Source: CAD feature listing. Evaluate the final solid. Frame: model axes, mm. Give positions to 0.01 mm unless a question says otherwise; leave off trailing zeros. Order: outer loops, then holes, each group sorted by start corner. A loop starts at its lowest first (then second) coordinate and runs counter-clockwise, first axis right, second up. Notation, with made-up numbers: (0, 71.5) -> (26, 71.5) arc R14 cw to (26, 79.5) -> close; hole circle Ø4 at (-36, 69.25). An arc over 180 degrees is marked (long way). Answer in a Markdown table with one row per item.
Autodesk Inventor part; units mm, degrees
ref_plane "YZ Plane" through (0, 0, 0) normal (1, 0, 0) x (0, 1, 0)
ref_plane "XZ Plane" through (0, 0, 0) normal (0, 1, 0) x (-1, 0, 0)
ref_plane "XY Plane" through (0, 0, 0) normal (0, 0, 1) x (1, 0, 0)
sketch "Skizze1" plane through (0, 0, 0) normal (0, 0, 1) x (1, 0, 0)
  line L0 (0, 78) -> (0, -13)
  line L1 (-15, 0) -> (90, 0)
  line L2 (0, 0) -> (75, 0)
  line L3 (75, 0) -> (75, 35)
  line L4 (75, 35) -> (0, 35)
  line L5 (0, 35) -> (0, 0)
  arc A0 (24, 35) -> (56, 35) centre (40, 65) ccw
  dimension "d0" = 75
  dimension "d1" = 35
  dimension "d3" = 35
  dimension "d4" = 30
  dimension "d6" = 34
extrude "Extrusion1" add sketch "Skizze1" along normal blind 2 contours L4 A0 L3 L1 L0
sketch "Skizze2" plane through (0, 0, 2) normal (0, 0, 1) x (1, 0, 0)
  line L0 (36, 6) -> (57, 6)
  line L1 (57, 6) -> (57, 27)
  line L2 (57, 27) -> (36, 27)
  line L3 (36, 27) -> (36, 6)
  line L4 (36, 6) -> (57, 27) construction
  line L5 (57, 6) -> (36, 27) construction
  line L6 (57, 27) -> (15, 27)
  line L7 (15, 27) -> (15, 6)
  line L8 (15, 6) -> (57, 6)
  line L9 (57, 6) -> (57, 27)
  line L10 (75, 0) -> (75, 35)
  line L11 (24, 35) -> (0, 35)
  circle A0 centre (61.35, 21.5) radius 2.25
  circle A1 centre (61.35, 11.5) radius 2.25
  circle A2 centre (11.85, 11.5) radius 2.25
  circle A3 centre (11.85, 21.5) radius 2.25
  point P0 (0, 0)
  point P1 (46.5, 16.5)
  dimension "d9" = 21
  dimension "d10" = 21
  dimension "d11" = 42
  dimension "d12" = 0
  dimension "d13" = 18
  dimension "d14" = 8
  dimension "d15" = 4.5
  dimension "d16" = 4.5
  dimension "d17" = 4.5
  dimension "d18" = 4.5
  dimension "d19" = 14.85
  dimension "d20" = 5
  dimension "d21" = 5
  dimension "d22" = 14.85
  dimension "d23" = 34.65
  dimension "d24" = 34.65
  dimension "d27" = 5
  dimension "d28" = 5
extrude "Extrusion2" cut sketch "Skizze2" against normal blind 2
sketch "Skizze3" plane through (0, 0, 2) normal (0, 0, 1) x (1, 0, 0)
  circle A0 centre (11.85, 21.5) radius 2.25
  circle A1 centre (61.35, 11.5) radius 2.25
  circle A2 centre (61.35, 21.5) radius 2.25
  circle A3 centre (11.85, 11.5) radius 2.25
  line L0 (15, 27) -> (15, 6)
  line L1 (15, 6) -> (57, 6)
  line L2 (57, 6) -> (57, 27)
  line L3 (57, 27) -> (15, 27)
  line L4 (0, 0) -> (0, 35)
  line L5 (0, 35) -> (24, 35)
  arc A4 (24, 35) -> (56, 35) centre (40, 65) ccw
  line L6 (56, 35) -> (75, 35)
  line L7 (75, 35) -> (75, 0)
  line L8 (75, 0) -> (0, 0)
  line L9 (75, 0) -> (75, 35)
  circle A5 centre (75, 17.5) radius 7
  line L10 (75, 0) -> (75, 35)
  dimension "d31" = 14
  dimension "d32" = 35
  dimension "d33" = 17.5
extrude "Extrusion3" add sketch "Skizze3" against normal blind 2 contours A5 L7 | L7 A5
sketch "Skizze4" plane through (0, 0, 2) normal (0, 0, 1) x (1, 0, 0)
  circle A0 centre (11.85, 21.5) radius 2.25
  circle A1 centre (61.35, 11.5) radius 2.25
  circle A2 centre (61.35, 21.5) radius 2.25
  circle A3 centre (11.85, 11.5) radius 2.25
  line L0 (15, 27) -> (15, 6)
  line L1 (15, 6) -> (57, 6)
  line L2 (57, 6) -> (57, 27)
  line L3 (57, 27) -> (15, 27)
  line L4 (0, 0) -> (0, 35)
  line L5 (0, 35) -> (24, 35)
  arc A4 (24, 35) -> (56, 35) centre (40, 65) ccw
  line L6 (56, 35) -> (75, 35)
  line L7 (75, 35) -> (75, 24.5)
  arc A5 (75, 10.5) -> (75, 24.5) centre (75, 17.5) ccw
  line L8 (75, 10.5) -> (75, 0)
  line L9 (75, 0) -> (0, 0)
  circle A6 centre (75, 17.5) radius 2.25
  dimension "d36" = 4.5
extrude "Extrusion4" cut sketch "Skizze4" against normal blind 2 contours A6
fillet "Rundung1" radius 15 1 edges at (0, 0, 1)
sketch "Skizze5" plane through (0, 0, 2) normal (0, 0, 1) x (1, 0, 0)
  line L0 (0, 35) -> (0, 15)
  circle A0 centre (0, 28) radius 7
  circle A1 centre (75, 17.5) radius 2.25
  arc A2 (75, 10.5) -> (75, 24.5) centre (75, 17.5) ccw
  line L1 (75, 10.5) -> (75, 0)
  line L2 (75, 0) -> (15, 0)
  arc A3 (0, 15) -> (15, 0) centre (15, 15) ccw
  line L3 (0, 15) -> (0, 35)
  line L4 (0, 35) -> (24, 35)
  arc A4 (24, 35) -> (56, 35) centre (40, 65) ccw
  line L5 (56, 35) -> (75, 35)
  line L6 (75, 35) -> (75, 24.5)
  circle A5 centre (11.85, 21.5) radius 2.25
  circle A6 centre (61.35, 11.5) radius 2.25
  circle A7 centre (61.35, 21.5) radius 2.25
  circle A8 centre (11.85, 11.5) radius 2.25
  line L7 (15, 27) -> (15, 6)
  line L8 (15, 6) -> (57, 6)
  line L9 (57, 6) -> (57, 27)
  line L10 (57, 27) -> (15, 27)
  circle A9 centre (0, 21) radius 7
  point P0 (0, 0)
  dimension "d40" = 14
  dimension "d46" = 14
extrude "Extrusion5" add sketch "Skizze5" against normal blind 2 contours A0 A9 L0 | L0 A9 A0 | A9 A0 L0 | L0 A0 A9 | A0 L0 A3 A9 | A0 A9 A3 L0
sketch "Skizze6" plane through (0, 0, 2) normal (0, 0, 1) x (1, 0, 0)
  circle A0 centre (75, 17.5) radius 2.25
  arc A1 (75, 10.5) -> (75, 24.5) centre (75, 17.5) ccw
  line L0 (75, 10.5) -> (75, 0)
  line L1 (75, 0) -> (15, 0)
  line L2 (0, 35) -> (24, 35)
  arc A2 (24, 35) -> (56, 35) centre (40, 65) ccw
  line L3 (56, 35) -> (75, 35)
  line L4 (75, 35) -> (75, 24.5)
  circle A3 centre (11.85, 21.5) radius 2.25
  circle A4 centre (61.35, 11.5) radius 2.25
  circle A5 centre (61.35, 21.5) radius 2.25
  circle A6 centre (11.85, 11.5) radius 2.25
  line L5 (15, 27) -> (15, 6)
  line L6 (15, 6) -> (57, 6)
  line L7 (57, 6) -> (57, 27)
  line L8 (57, 27) -> (15, 27)
  circle A7 centre (0, 28) radius 2.25
  circle A8 centre (75, 17.5) radius 75.7314
  circle A9 centre (-0.7298, 18) radius 7
  arc A10 (0.0334, 14.0001) -> (15, 0) centre (15, 15) ccw
  arc A11 (-6.0622, 24.5) -> (0.0334, 14.0001) centre (0, 21) ccw
  arc A12 (0, 35) -> (-6.0622, 24.5) centre (0, 28) ccw
  point P0 (0, 0)
  point P1 (0, 21)
  dimension "d43" = 4.5
  dimension "d47" = 14
  dimension "d48" = 3
extrude "Extrusion6" cut sketch "Skizze6" against normal blind 2 contours A8 A7 | A7 A8
fillet "Rundung2" radius 15 2 edges at (-6.0622, 24.5, 1) (0.0334, 14.0001, 1)
sketch "Skizze7" plane through (0, 0, 2) normal (0, 0, 1) x (1, 0, 0)
  circle A0 centre (0, 28) radius 2.25
  circle A1 centre (75, 17.5) radius 2.25
  arc A2 (75, 10.5) -> (75, 24.5) centre (75, 17.5) ccw
  line L0 (75, 10.5) -> (75, 0)
  line L1 (75, 0) -> (15, 0)
  arc A3 (1.286, 8.9233) -> (15, 0) centre (15, 15) ccw
  arc A4 (1.286, 8.9233) -> (-3.9544, 15.2239) centre (-12.428, 2.8466) ccw
  arc A5 (-6.9108, 22.1136) -> (-3.9544, 15.2239) centre (0, 21) ccw
  arc A6 (-6.9108, 22.1136) -> (-6.9108, 26.8864) centre (-21.7198, 24.5) ccw
  arc A7 (0, 35) -> (-6.9108, 26.8864) centre (0, 28) ccw
  line L2 (0, 35) -> (24, 35)
  arc A8 (24, 35) -> (56, 35) centre (40, 65) ccw
  line L3 (56, 35) -> (75, 35)
  line L4 (75, 35) -> (75, 24.5)
  circle A9 centre (11.85, 21.5) radius 2.25
  circle A10 centre (61.35, 11.5) radius 2.25
  circle A11 centre (61.35, 21.5) radius 2.25
  circle A12 centre (11.85, 11.5) radius 2.25
  line L5 (15, 27) -> (15, 6)
  line L6 (15, 6) -> (57, 6)
  line L7 (57, 6) -> (57, 27)
  line L8 (57, 27) -> (15, 27)
  arc A13 (75, 10.5) -> (75, 24.5) centre (75, 17.5) ccw
  circle A14 centre (75, 17.5) radius 75.7314
  circle A15 centre (-0.7166, 19) radius 2.25
  point P0 (0, 0)
  dimension "d50" = 9
  dimension "d51" = 4.5
extrude "Extrusion7" cut sketch "Skizze7" against normal blind 2 contours A15 A14 | A14 A15
fillet "Rundung3" radius 15 4 edges at (75, 35, 1) (56, 35, 1) (24, 35, 1) (75, 0, 1)
sketch "Skizze8" plane through (0, 0, 2) normal (0, 0, 1) x (1, 0, 0)
  circle A0 centre (-0.7166, 19) radius 2.25
  arc A1 (1.286, 8.9233) -> (-3.9544, 15.2239) centre (-12.428, 2.8466) ccw
  arc A2 (-6.9108, 22.1136) -> (-3.9544, 15.2239) centre (0, 21) ccw
  arc A3 (-6.9108, 22.1136) -> (-6.9108, 26.8864) centre (-21.7198, 24.5) ccw
  arc A4 (0, 35) -> (-6.9108, 26.8864) centre (0, 28) ccw
  line L0 (0, 35) -> (20.6093, 35)
  arc A5 (26.5452, 33.7755) -> (20.6093, 35) centre (20.6093, 20) ccw
  arc A6 (26.5452, 33.7755) -> (53.4548, 33.7755) centre (40, 65) ccw
  arc A7 (59.3907, 35) -> (53.4548, 33.7755) centre (59.3907, 20) ccw
  line L1 (59.3907, 35) -> (60.6909, 35)
  arc A8 (75, 24.5) -> (60.6909, 35) centre (60.6909, 20) ccw
  arc A9 (75, 10.5) -> (75, 24.5) centre (75, 17.5) ccw
  arc A10 (60.6909, 0) -> (75, 10.5) centre (60.6909, 15) ccw
  line L2 (60.6909, 0) -> (15, 0)
  arc A11 (1.286, 8.9233) -> (15, 0) centre (15, 15) ccw
  circle A12 centre (0, 28) radius 2.25
  circle A13 centre (75, 17.5) radius 2.25
  circle A14 centre (11.85, 21.5) radius 2.25
  circle A15 centre (61.35, 11.5) radius 2.25
  circle A16 centre (61.35, 21.5) radius 2.25
  circle A17 centre (11.85, 11.5) radius 2.25
  line L3 (15, 27) -> (15, 6)
  line L4 (15, 6) -> (57, 6)
  line L5 (57, 6) -> (57, 27)
  line L6 (57, 27) -> (15, 27)
  circle A18 centre (75, 17.5) radius 2.25
  circle A19 centre (75, 17.5) radius 82.0816
  line L7 (-6.8487, 11.3205) -> (6.8192, 2.4272)
  arc A20 (1.286, 8.9233) -> (15, 0) centre (15, 15) ccw
  line L8 (6.8192, 2.4272) -> (-0.8956, 15)
  line L9 (-0.8956, 15) -> (-5.8598, 18.2396)
  line L10 (-5.8598, 18.2396) -> (-6.9924, 21.3263)
  arc A21 (-6.9108, 22.1136) -> (-3.9544, 15.2239) centre (0, 21) ccw
  point P0 (0, 0)
extrude "Extrusion8" add sketch "Skizze8" against normal blind 2 contours A11 L7 A19 A2 A1 | A1 A2 L10 L9 L8 A11
fillet "Rundung4" radius 5 1 edges at (-6.8487, 11.3205, 1)
sketch "Skizze9" plane through (0, 0, 2) normal (0, 0, 1) x (1, 0, 0)
  arc A0 (26.5452, 33.7755) -> (20.6093, 35) centre (20.6093, 20) ccw
  arc A1 (26.5452, 33.7755) -> (53.4548, 33.7755) centre (40, 65) ccw
  arc A2 (59.3907, 35) -> (53.4548, 33.7755) centre (59.3907, 20) ccw
  line L0 (59.3907, 35) -> (60.6909, 35)
  arc A3 (75, 24.5) -> (60.6909, 35) centre (60.6909, 20) ccw
  arc A4 (75, 10.5) -> (75, 24.5) centre (75, 17.5) ccw
  arc A5 (60.6909, 0) -> (75, 10.5) centre (60.6909, 15) ccw
  line L1 (60.6909, 0) -> (15, 0)
  arc A6 (6.8192, 2.4272) -> (15, 0) centre (15, 15) ccw
  line L2 (6.8192, 2.4272) -> (-4.7351, 9.9453)
  arc A7 (-7.0034, 13.918) -> (-4.7351, 9.9453) centre (-2.0082, 14.1362) ccw
  arc A8 (-6.9924, 21.3263) -> (-7.0034, 13.918) centre (75, 17.5) ccw
  arc A9 (-6.9108, 22.1136) -> (-6.9924, 21.3263) centre (0, 21) ccw
  arc A10 (-6.9108, 22.1136) -> (-6.9108, 26.8864) centre (-21.7198, 24.5) ccw
  arc A11 (0, 35) -> (-6.9108, 26.8864) centre (0, 28) ccw
  line L3 (0, 35) -> (20.6093, 35)
  circle A12 centre (-0.7166, 19) radius 2.25
  circle A13 centre (0, 28) radius 2.25
  circle A14 centre (75, 17.5) radius 2.25
  circle A15 centre (11.85, 21.5) radius 2.25
  circle A16 centre (61.35, 11.5) radius 2.25
  circle A17 centre (61.35, 21.5) radius 2.25
  circle A18 centre (11.85, 11.5) radius 2.25
  line L4 (15, 27) -> (15, 6)
  line L5 (15, 6) -> (57, 6)
  line L6 (57, 6) -> (57, 27)
  line L7 (57, 27) -> (15, 27)
  point P0 (0, 0)
extrude "Extrusion9" add sketch "Skizze9" against normal up to surface (2 mm away) contours A12
sketch "Skizze10" plane through (0, 0, 2) normal (0, 0, 1) x (1, 0, 0)
  arc A0 (26.5452, 33.7755) -> (20.6093, 35) centre (20.6093, 20) ccw
  arc A1 (26.5452, 33.7755) -> (53.4548, 33.7755) centre (40, 65) ccw
  arc A2 (59.3907, 35) -> (53.4548, 33.7755) centre (59.3907, 20) ccw
  line L0 (59.3907, 35) -> (60.6909, 35)
  arc A3 (75, 24.5) -> (60.6909, 35) centre (60.6909, 20) ccw
  arc A4 (75, 10.5) -> (75, 24.5) centre (75, 17.5) ccw
  arc A5 (60.6909, 0) -> (75, 10.5) centre (60.6909, 15) ccw
  line L1 (60.6909, 0) -> (15, 0)
  arc A6 (6.8192, 2.4272) -> (15, 0) centre (15, 15) ccw
  line L2 (6.8192, 2.4272) -> (-4.7351, 9.9453)
  arc A7 (-7.0034, 13.918) -> (-4.7351, 9.9453) centre (-2.0082, 14.1362) ccw
  arc A8 (-6.9924, 21.3263) -> (-7.0034, 13.918) centre (75, 17.5) ccw
  arc A9 (-6.9108, 22.1136) -> (-6.9924, 21.3263) centre (0, 21) ccw
  arc A10 (-6.9108, 22.1136) -> (-6.9108, 26.8864) centre (-21.7198, 24.5) ccw
  arc A11 (0, 35) -> (-6.9108, 26.8864) centre (0, 28) ccw
  line L3 (0, 35) -> (20.6093, 35)
  circle A12 centre (0, 28) radius 2.25
  circle A13 centre (75, 17.5) radius 2.25
  circle A14 centre (11.85, 21.5) radius 2.25
  circle A15 centre (61.35, 11.5) radius 2.25
  circle A16 centre (61.35, 21.5) radius 2.25
  circle A17 centre (11.85, 11.5) radius 2.25
  line L4 (15, 27) -> (15, 6)
  line L5 (15, 6) -> (57, 6)
  line L6 (57, 6) -> (57, 27)
  line L7 (57, 27) -> (15, 27)
  circle A18 centre (75, 17.5) radius 75.7314
  circle A19 centre (-0.6505, 14) radius 2.25
  point P0 (0, 0)
  dimension "d60" = 14
  dimension "d61" = 4.5
extrude "Extrusion10" cut sketch "Skizze10" against normal blind 2 contours A19 A18 | A18 A19
equation "\"d16\" = d15"
equation "\"d17\" = d15"
equation "\"d18\" = d17"
equation "\"d33\" = 0.5 * d32"
properties part number "Adapter"
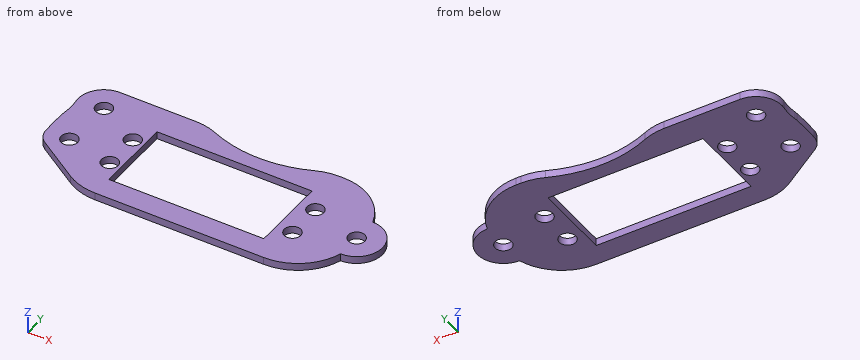
(1) First-contact query: pin 1 Ø0.6 at (y, z) = (14, 1) entering from -X; pin 2 Ø4 at (x, y) = (11.85, 11.5) entering from +Z; pin 3 Ø1 at (y, z) = (8.5, 0.5) entering from +X; pin 4 Ø0.6 at (x, z) = (32, 1.5) entering from +Y. Flat tips, straight axial feed; report the tip coordinate or a pass-through.
A:
| item | result |
|---|---|
| pin 1 | stops at x = -7.02 |
| pin 2 | passes through |
| pin 3 | stops at x = 74.44 |
| pin 4 | stops at y = 32.03 |
(2) Section query B-B (x = 11.85). Return the cut outline in (y, z), plus the area to 3 significant figures.
A:
| item | result |
|---|---|
| outline | (0.33, 0) -> (9.25, 0) -> (9.25, 2) -> (0.33, 2) -> close; (13.75, 0) -> (19.25, 0) -> (19.25, 2) -> (13.75, 2) -> close; (23.75, 0) -> (35, 0) -> (35, 2) -> (23.75, 2) -> close |
| area | 51.3 mm^2 |
(3) Section query A-A (x = 22). Return the cut outline in (y, z), plus the area to 3 significant figures.
A:
| item | result |
|---|---|
| outline | (0, 0) -> (6, 0) -> (6, 2) -> (0, 2) -> close; (27, 0) -> (34.94, 0) -> (34.94, 2) -> (27, 2) -> close |
| area | 27.9 mm^2 |
(4) Section query C-C (x = 54.5). Return the cut outline in (y, z), plus the area to 3 significant figures.
A:
| item | result |
|---|---|
| outline | (0, 0) -> (6, 0) -> (6, 2) -> (0, 2) -> close; (27, 0) -> (34.18, 0) -> (34.18, 2) -> (27, 2) -> close |
| area | 26.4 mm^2 |
(5) Section query D-D (z = 1.35). Give the number of separate pieces and of enclosed holes in the cut face, plus the area to 3 significant figures.
A:
| item | result |
|---|---|
| separate pieces | 1 |
| enclosed holes | 8 |
| area | 1,670 mm^2 |
(6) Ray query, probe 1 along Y at (x, z) = (61.35, 0.9); probe 2 along X at (y, z) = (14, 0.4); probe 3 along Y at (x, z) = (59.5, 0.25). Return the intervals inside material, ascending.
A:
| item | result |
|---|---|
| probe 1 | y = 0.01 to 9.25, 13.75 to 19.25, 23.75 to 34.99 |
| probe 2 | x = -7.01 to -2.9, 1.6 to 15, 57 to 81.06 |
| probe 3 | y = 0 to 10.22, 12.78 to 20.22, 22.78 to 35 |
